Geometry: final body of the model. Coordinates: model frame, mm. Face numbers are marked on the shaded views. A direction names the side the tool comes from. Give positions to 0.01 mm unless a question says otherwise; leave off trailing zeros. Write each loop counter-clockwise with the first axis right and the second up, starting at its lowest first coordinate (ties: lowest second). Pieces come first, ordered by that corner, then holes. Notation, with made-up numbers: (17, 18.5) - (61, 18.5) arc R17 cw to (61, 30.5) - close; hole circle Ø1 at (-34.5, -19). An arc over 180 degrees is marked (long way). Return JSON: item names as keys, results as strings.
from build123d import *

# Parameters (mm, degrees)
EXTRUDE_1_DEPTH      = 29
CUT_EXTRUDE_1_DEPTH  = 8
EXTRUDE_3_DEPTH      = 5
EXTRUDE_4_DEPTH      = 5
EXTRUDE_7_DEPTH      = 5
EXTRUDE_8_DEPTH      = 5
CUT_EXTRUDE_2_DEPTH  = 8
CUT_EXTRUDE_3_DEPTH  = 8
CUT_EXTRUDE_4_DEPTH  = 8
CUT_EXTRUDE_5_DEPTH  = 8
EXTRUDE_9_DEPTH      = 4
EXTRUDE_9_DEPTH_BACK = 15
CUT_EXTRUDE_6_DEPTH  = 123.591294734
EXTRUDE_10_DEPTH     = 12
CUT_EXTRUDE_7_DEPTH  = 10
CUT_EXTRUDE_8_REACH  = 131.356
SKETCH_19_R          = 4
SKETCH_19_R_2        = 0.75
CUT_EXTRUDE_9_REACH  = 128.701
SKETCH_20_R          = 1.459599559
SKETCH_20_R_2        = 1.556195018
SKETCH_20_R_3        = 1.5


with BuildPart() as part:
    # 草图1 → 凸台-拉伸1 (new, symmetric)
    with BuildSketch(Plane.XY):
        Polygon((0, 0), (25, 0), (27.537171242, 29), (25, 58), (15, 58), (15, 23), (0, 8), align=None)
    extrude(amount=EXTRUDE_1_DEPTH, both=True)

    # 草图2 → 切除-拉伸1 (cut)
    with BuildSketch(Plane.ZY.offset(-15)):
        Polygon((-27, 58), (-27, 55.814681899), (-13.451752106, 57), (0.148247894, 57), (13.696495788, 55.814681899), (27.089881229, 53.453066682), (27.089881229, 58), align=None)
    extrude(amount=-CUT_EXTRUDE_1_DEPTH, mode=Mode.SUBTRACT)

    # 草图3 → 凸台-拉伸3 (add, symmetric)
    with BuildSketch(Plane(origin=(15, 56.407340949, -20.225876053), x_dir=(1, 0, 0), z_dir=(0, 0.08715574274765847, 0.9961946980917457))):
        Polygon((-9.323445702, 54.044998978), (-8.171455002, 46.660954361), (-4.917561857, 39.352590699), (0, 21), (0, 0), (8, 0), (6.465357578, 21.946409106), (-0.046005512, 40.856780618), (-7.557550516, 54.983942103), align=None)
    extrude(amount=EXTRUDE_3_DEPTH, both=True)

    # 草图4 → 凸台-拉伸4 (add, symmetric)
    with BuildSketch(Plane(origin=(15, 57, -6.651752106), x_dir=(1, 0, 0), z_dir=(0, 0, 1))):
        Polygon((0, 0), (8, 0), (6.395601104, 22.943973156), (-0.44133014, 42.799863244), (-8.422346707, 57.809972322), (-10.188241893, 56.871029197), (-8.633642368, 49.083652916), (-5.176380902, 41.318516526), (0, 22), align=None)
    extrude(amount=EXTRUDE_4_DEPTH, both=True)

    # 草图5 → 凸台-拉伸7 (add, symmetric)
    with BuildSketch(Plane(origin=(15, 56.407340949, 6.922371841), x_dir=(1, 0, 0), z_dir=(0, -0.08715574274765847, 0.9961946980917457))):
        Polygon((0, 0), (8, 0), (6.465357578, 21.946409106), (-0.046005512, 40.856780618), (-7.557550516, 54.983942103), (-9.323445702, 54.044998978), (-8.171455002, 46.660954361), (-4.917561857, 39.352590699), (0, 21), align=None)
    extrude(amount=EXTRUDE_7_DEPTH, both=True)

    # 草图6 → 凸台-拉伸8 (add, symmetric)
    with BuildSketch(Plane(origin=(15, 54.63387429, 20.393188509), x_dir=(1, 0, 0), z_dir=(0, -0.17364817766693064, 0.9848077530122081))):
        Polygon((0, 0), (8, 0), (6.535114051, 20.948845055), (0.674887271, 37.968179416), (-6.367186171, 51.212393309), (-8.133081356, 50.273450184), (-7.45044859, 43.272329979), (-4.399923767, 36.420739047), (0, 20), align=None)
    extrude(amount=EXTRUDE_8_DEPTH, both=True)

    # 草图9 → 切除-拉伸2 (cut)
    with BuildSketch(Plane(origin=(43.786407244, 15.019497062, -1.314035725), x_dir=(-0.027653196730496193, -0.006835672416694662, -0.9995942048117308), z_dir=(0.945518575599319, 0.32432926933772815, -0.028375134316697356))):
        Polygon((16.019101355, 67.443389025), (18.714253027, 87.286175055), (21.05291991, 102.947141542), (27.031237201, 102.437511905), (26.685342748, 86.606668873), (25.982963507, 66.594006296), (29.629783933, 109.373797793), (19.665921781, 110.223180522), align=None)
    extrude(amount=-CUT_EXTRUDE_2_DEPTH, mode=Mode.SUBTRACT)

    # 草图10 → 切除-拉伸3 (cut)
    with BuildSketch(Plane(origin=(43.736994655, 15.059854982, 0), x_dir=(0, 0, -1), z_dir=(0.9455185755993187, 0.32556815445715115, 0))):
        Polygon((1.651752106, 68.622785261), (2.651752106, 89.622785261), (3.651752106, 106.413487051), (9.651752106, 106.413487051), (10.651752106, 89.622785261), (11.651752106, 68.622785261), (11.651752106, 115.571899367), (1.651752106, 115.571899367), align=None)
    extrude(amount=-CUT_EXTRUDE_3_DEPTH, mode=Mode.SUBTRACT)

    # 草图11 → 切除-拉伸4 (cut)
    with BuildSketch(Plane(origin=(43.429484648, 14.897066422, 1.303324432), x_dir=(0.02765319673049623, 0.006835672416694678, -0.9995942048117308), z_dir=(0.9455185755993187, 0.32432926933772854, 0.028375134316697394))):
        Polygon((-12.684857793, 66.627338038), (-13.387237034, 86.640000614), (-13.733131487, 102.470843646), (-7.754814196, 102.980473283), (-5.416147313, 87.319506797), (-2.720995641, 67.476720766), (-6.546649191, 112.354351713), (-16.478235605, 111.126351676), align=None)
    extrude(amount=-CUT_EXTRUDE_4_DEPTH, mode=Mode.SUBTRACT)

    # 草图12 → 切除-拉伸5 (cut)
    with BuildSketch(Plane(origin=(43.353791536, 14.701119108, 2.592203945), x_dir=(0.05512742044977168, 0.013471340172277213, -0.9983884467022428), z_dir=(0.9455185755993187, 0.32062204264327854, 0.0565343167278701))):
        Polygon((-26.718901534, 63.408631661), (-28.781224347, 81.318037698), (-30.304296285, 96.088755689), (-24.390936546, 97.104716612), (-20.896744695, 82.672652262), (-16.863301969, 65.101899866), (-23.990371814, 106.58472359), (-33.845971379, 104.891455385), align=None)
    extrude(amount=-CUT_EXTRUDE_5_DEPTH, mode=Mode.SUBTRACT)

    # 草图13 → 凸台-拉伸9 (add, two sides: drawn at the far end of the back side and taken through both)
    with BuildSketch(Plane(origin=(0, 0, -29), x_dir=(-1, 0, 0), z_dir=(0, 0, -1)).offset(-EXTRUDE_9_DEPTH_BACK)):
        Polygon((-15, 42), (-21, 36), (-21, 0), (0, 0), (0, 27), align=None)
    extrude(amount=EXTRUDE_9_DEPTH + EXTRUDE_9_DEPTH_BACK)

    # 草图14 → 切除-拉伸6 (cut, through all)
    with BuildSketch(Plane.XZ):
        Polygon((21, -29), (3, -33), (0, -30), (0, -35.356420502), (21, -35.356420502), (21, -33), align=None)
    extrude(amount=-CUT_EXTRUDE_6_DEPTH, mode=Mode.SUBTRACT)

    # 草图17 → 凸台-拉伸10 (add)
    with BuildSketch(Plane(origin=(9.583983071, 5.668293949, 2.129774016), x_dir=(-0.4880935300919712, 0.8660254037844418, -0.10846522890932642), z_dir=(-0.845402792964955, -0.4999999999999946, -0.18786728732554522))):
        Polygon((28.095834077, 32.86496436), (43.684291345, 41.86496436), (54.517176629, 43.775094314), (63.782054485, 47.744457312), (63.607743, 49.736846708), (41.691459642, 47.819420367), (21.752688327, 38.521818609), (16.095834077, 32.86496436), align=None)
    extrude(amount=-EXTRUDE_10_DEPTH)

    # 草图18 → 切除-拉伸7 (cut)
    with BuildSketch(Plane(origin=(11.38136915, -3.321366881, -42.376498538), x_dir=(-0.9659724085627504, -0.020280380390013637, -0.25784881629884493), z_dir=(0.2586451260790556, -0.07547908730517995, -0.9630190061131331))):
        Polygon((1.682136929, 51.286517247), (14.512238635, 69.331973467), (20.638759875, 65.945863974), (12.184744769, 45.481758116), (26.51939396, 71.417580015), (15.357154401, 76.028860982), align=None)
    extrude(amount=-CUT_EXTRUDE_7_DEPTH, mode=Mode.SUBTRACT)

    # 切除-拉伸8: up to this plane
    cut_extrude_8_end = Plane(origin=(15, 23, 29), z_dir=(0.7071067811865438, -0.7071067811865512, 0))
    # 草图19 → 切除-拉伸8 (cut, up to the surface)
    with BuildSketch(Plane.XZ, mode=Mode.PRIVATE) as cut_extrude_8_sk1:
        with Locations(Location((9, 0, 0), (0, 0, 270))):
            Circle(SKETCH_19_R)
    cut_extrude_8_tool1 = split(extrude(cut_extrude_8_sk1.sketch, amount=-CUT_EXTRUDE_8_REACH, mode=Mode.PRIVATE), bisect_by=cut_extrude_8_end, keep=Keep.BOTH, mode=Mode.PRIVATE)
    add(cut_extrude_8_tool1.solids().sort_by_distance((9, 0, 0))[0], mode=Mode.SUBTRACT)
    # 草图19 → 切除-拉伸8 (cut, up to the surface)
    with BuildSketch(Plane.XZ, mode=Mode.PRIVATE) as cut_extrude_8_sk2:
        with Locations(Location((2.2, 0, 0), (0, 0, 270))):
            Circle(SKETCH_19_R_2)
    cut_extrude_8_tool2 = split(extrude(cut_extrude_8_sk2.sketch, amount=-CUT_EXTRUDE_8_REACH, mode=Mode.PRIVATE), bisect_by=cut_extrude_8_end, keep=Keep.BOTH, mode=Mode.PRIVATE)
    add(cut_extrude_8_tool2.solids().sort_by_distance((2.2, 0, 0))[0], mode=Mode.SUBTRACT)
    # 草图19 → 切除-拉伸8 (cut, up to the surface)
    with BuildSketch(Plane.XZ, mode=Mode.PRIVATE) as cut_extrude_8_sk3:
        with Locations(Location((9, 6.8, 0), (0, 0, 270))):
            Circle(SKETCH_19_R_2)
    cut_extrude_8_tool3 = split(extrude(cut_extrude_8_sk3.sketch, amount=-CUT_EXTRUDE_8_REACH, mode=Mode.PRIVATE), bisect_by=cut_extrude_8_end, keep=Keep.BOTH, mode=Mode.PRIVATE)
    add(cut_extrude_8_tool3.solids().sort_by_distance((9, 0, 6.8))[0], mode=Mode.SUBTRACT)
    # 草图19 → 切除-拉伸8 (cut, up to the surface)
    with BuildSketch(Plane.XZ, mode=Mode.PRIVATE) as cut_extrude_8_sk4:
        with Locations(Location((9, -6.8, 0), (0, 0, 270))):
            Circle(SKETCH_19_R_2)
    cut_extrude_8_tool4 = split(extrude(cut_extrude_8_sk4.sketch, amount=-CUT_EXTRUDE_8_REACH, mode=Mode.PRIVATE), bisect_by=cut_extrude_8_end, keep=Keep.BOTH, mode=Mode.PRIVATE)
    add(cut_extrude_8_tool4.solids().sort_by_distance((9, 0, -6.8))[0], mode=Mode.SUBTRACT)

    # 切除-拉伸9: up to this plane
    cut_extrude_9_end = Plane(origin=(15, 23, 29), z_dir=(0.7071067811865438, -0.7071067811865512, 0))
    # 草图20 → 切除-拉伸9 (cut, up to the surface)
    with BuildSketch(Plane(origin=(0, 3, 0), x_dir=(-1, 0, 0), z_dir=(0, -1, 0)), mode=Mode.PRIVATE) as cut_extrude_9_sk1:
        with Locations(Location((-9, 6.8, 0), (0, 0, 90))):
            Circle(SKETCH_20_R)
    cut_extrude_9_tool1 = split(extrude(cut_extrude_9_sk1.sketch, amount=-CUT_EXTRUDE_9_REACH, mode=Mode.PRIVATE), bisect_by=cut_extrude_9_end, keep=Keep.BOTH, mode=Mode.PRIVATE)
    add(cut_extrude_9_tool1.solids().sort_by_distance((9, 3, -6.8))[0], mode=Mode.SUBTRACT)
    # 草图20 → 切除-拉伸9 (cut, up to the surface)
    with BuildSketch(Plane(origin=(0, 3, 0), x_dir=(-1, 0, 0), z_dir=(0, -1, 0)), mode=Mode.PRIVATE) as cut_extrude_9_sk2:
        with Locations(Location((-2.2, 0, 0), (0, 0, 90))):
            Circle(SKETCH_20_R_2)
    cut_extrude_9_tool2 = split(extrude(cut_extrude_9_sk2.sketch, amount=-CUT_EXTRUDE_9_REACH, mode=Mode.PRIVATE), bisect_by=cut_extrude_9_end, keep=Keep.BOTH, mode=Mode.PRIVATE)
    add(cut_extrude_9_tool2.solids().sort_by_distance((2.2, 3, 0))[0], mode=Mode.SUBTRACT)
    # 草图20 → 切除-拉伸9 (cut, up to the surface)
    with BuildSketch(Plane(origin=(0, 3, 0), x_dir=(-1, 0, 0), z_dir=(0, -1, 0)), mode=Mode.PRIVATE) as cut_extrude_9_sk3:
        with Locations(Location((-9, -6.8, 0), (0, 0, 90))):
            Circle(SKETCH_20_R_3)
    cut_extrude_9_tool3 = split(extrude(cut_extrude_9_sk3.sketch, amount=-CUT_EXTRUDE_9_REACH, mode=Mode.PRIVATE), bisect_by=cut_extrude_9_end, keep=Keep.BOTH, mode=Mode.PRIVATE)
    add(cut_extrude_9_tool3.solids().sort_by_distance((9, 3, 6.8))[0], mode=Mode.SUBTRACT)


solid = part.part
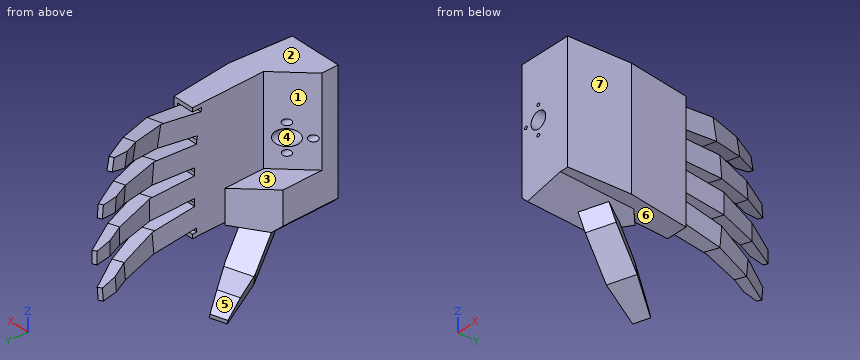
Q1. Section query A-A, the plane y = 70. Return the cut outline in (x, z), plus the area to 3 significant figures.
Answer key:
{"outline": "(15, -26.43) - (22.02, -26.43) - (22.08, -16.4) - (15, -16.4) - close; (15, -11.65) - (22.09, -11.65) - (22.09, -1.65) - (15, -1.65) - close; (15, 3.09) - (22.08, 3.09) - (22.02, 13.13) - (15, 13.13) - close; (15, 18.03) - (21.97, 18.03) - (21.85, 28.18) - (15, 28.18) - close", "area": "283 mm^2"}
Q2. Pin query (flat end, axial travel): P1, Ø1.4, axis at x = 19.5, y = 56, coming from the -Z side; P2, Ø4, axis at y = 53, z = -3.5, coming from the +X side; P3, Ø1.5, axis at x = 0, z = -44, coming from the -Y side. Return the tip coordinate at first contact, or that it passes through.
Answer key:
{"P1": "stops at z = -29", "P2": "stops at x = 25.61", "P3": "stops at y = 37.91"}
Q3. Mould query, pull axis X, two halves, no side actions, for the marked faces 4, 5, 6 and 7. Classes: pulls with the +X half, pulls with the -X half, needs draft (parallel to the pull), parting line crosses it, or undercut.
Answer key:
{"face 4": "undercut", "face 5": "pulls with the -X half", "face 6": "needs draft", "face 7": "pulls with the +X half"}
Q4. Material intervals for probe 1 along X at (y, z) = (2.15, 0); probe 2 along Z at (x, y) = (9, 6.25); probe 3 along Z at (x, y) = (16, 65.5), sorted ascending. Write a range as [from, to].
Answer key:
{"probe 1": "x = [0, 1.45], [2.95, 5], [13, 25.19]", "probe 2": "z = [-31.67, -8.26], [-5.34, -4], [4, 5.3], [8.3, 29]", "probe 3": "z = [-26.04, -16], [-11.65, -1.65], [2.7, 12.74], [17.23, 27.39]"}
Q5. Section query B-B, the plane y = 51. Return the cut outline in (x, z).
Answer key:
{"outline": "(-5.35, -45.53) - (-4.12, -50.8) - (7.5, -47.68) - (6.28, -41.85) - close; (15, -29) - (25.61, -29) - (25.61, 29) - (15, 29) - close"}
Q6. Set-up query: the marked faces 1, 2 and 3. Return all of +Z, -Z, +X, -X, +Y, -Y with unobstructed straight access to the full face (end or side cutting, diameter ignored); none if empty.
Answer key:
{"face 1": "+Z, -X", "face 2": "+Z, +X, -X, -Y", "face 3": "+Z, -X, +Y"}
